Geometry check sheet. Reference: the model listing, model coordinates, mm. A direction names the side the tool comes from. Give positions to 0.01 mm unless a question says otherwise; leave off trailing zeros. Write each loop counter-clockwise with the first axis right and the second up, starting at its lowest first coordinate (ties: lowest second). Pieces come first, ordered by that corner, then holes.
(1) Mould release check, pull along Y, two halves, no side actions. Record for faces 5 (the flat face through (0, -8.9, 3)), 6 (the flat face through (22, 10, -12)), 7 (the flat face through (19, 20, -11)), 8 (the cylindrical face through (9.6, -11, 2.5)): +Y half, -Y half, draft (parallel to the pull), parting line (faces both ways), or undercut.
(2) Tool access check on faces 1 (the flat face through (0, -20, 2)), 2 (the flat face through (15, 2, 2)), 3 (the flat face through (0, -13.1, 3)), 4 (the flat face through (0, -5, 0)). Record the directions out of +Z, -Z, +X, -X, +Y, -Y that give a thin tool (end or side, any length) a straight path to the whole face; none if there is none.
(3) Cross-section at A-A (y = -11). Record the boundary of the cut face in (x, z), and give its area (3 significant figures).
(4) Cross-section at C-C (x = 28). Record the boundary of the cut face in (y, z), and give its area (3 significant figures).
(5) Thickness scan on line 1 along Y through (x, z) = (7, 2.5); line 2 along Z through (x, y) = (-9, -9); line 3 along X through (y, z) = (10, 3.5). Record the ranges inside material, lowest first.
(6) Cross-section at D-D (z = -24). Record the boundary of the cut face in (x, y), and give its area (3 significant figures).
(7) Cross-section at B-B (y = 13). Record the boundary of the cut face in (x, z), and give its area (3 significant figures).
(8) Depth check by flat-ended pin: P1, Ø1.5, axis at y = 6, z = 3.5, coming from the +X side; P2, Ø5, axis at x = 42.5, y = 14.5, coming from the -Z side; P3, Ø12, axis at x = 36, y = 11.5, coming from the -Z side. Enter the tip coordinate at first touch or a pass-through.
```python
from build123d import *

# Parameters (mm, degrees)
SKETCH1_W           = 30
SKETCH1_H           = 40
BOSS_EXTRUDE1_DEPTH = 5
BOSS_EXTRUDE2_DEPTH = 10
FILLET2_R           = 5
CUT_EXTRUDE1_DEPTH  = 10


with BuildPart() as part:
    # Sketch1 → Boss-Extrude1 (new body)
    with BuildSketch(Plane.XY):
        Rectangle(SKETCH1_W, SKETCH1_H)
    extrude(amount=BOSS_EXTRUDE1_DEPTH)

    # Sketch2 → Boss-Extrude2 (add)
    with BuildSketch(Plane(origin=(0, 20, 0), x_dir=(1, 0, 0), z_dir=(0, 1, 0))):
        Polygon((-15, 0), (64.346756059, 37), (15, 0), align=None)
    extrude(amount=-BOSS_EXTRUDE2_DEPTH)

    # Fillet2
    fillet2_edges = [part.edges().sort_by_distance(p)[0] for p in [
        (15, -20, 2.5),
        (-15, -20, 2.5),
    ]]
    fillet(fillet2_edges, radius=FILLET2_R)

    # Sketch4 → Cut-Extrude1 (cut)
    with BuildSketch(Plane.XY.offset(5)):
        with BuildLine():
            Line((7.5, -13.1), (-7.5, -13.1))
            ThreePointArc((-7.5, -13.1), (-9.6, -11), (-7.5, -8.9))
            Line((-7.5, -8.9), (7.5, -8.9))
            ThreePointArc((7.5, -8.9), (9.6, -11), (7.5, -13.1))
        make_face()
    extrude(amount=-CUT_EXTRUDE1_DEPTH, mode=Mode.SUBTRACT)


solid = part.part
```
Reply:
1. face 5: undercut
1. face 6: -Y half
1. face 7: +Y half
1. face 8: undercut
2. face 1: +Z, -Z, +X, -X, -Y
2. face 2: +Z, +X, +Y, -Y
2. face 3: +Z, -Z
2. face 4: -Z, +X, -X, -Y
3. outline: (-15, 0) - (-9.6, 0) - (-9.6, 5) - (-15, 5) - close; (9.6, 0) - (15, 0) - (15, 5) - (9.6, 5) - close
3. area: 54.0 mm2
4. outline: (10, -20.05) - (20, -20.05) - (20, -9.75) - (10, -9.75) - close
4. area: 103 mm2
5. line 1: y = -20 to -13.1, -8.9 to 20
5. line 2: z = 0 to 5
5. line 3: x = -15 to 15
6. outline: (36.47, 10) - (47.01, 10) - (47.01, 20) - (36.47, 20) - close
6. area: 105 mm2
7. outline: (-15, 0) - (64.35, -37) - (15, 0) - (15, 5) - (-15, 5) - close
7. area: 705 mm2
8. P1: stops at x = 15
8. P2: stops at z = -27.98
8. P3: stops at z = -26.58
